Autodesk Inventor part; units mm, degrees
ref_plane "YZ Plane" through (0, 0, 0) normal (1, 0, 0) x (0, 1, 0)
ref_plane "XZ Plane" through (0, 0, 0) normal (0, 1, 0) x (-1, 0, 0)
ref_plane "XY Plane" through (0, 0, 0) normal (0, 0, 1) x (1, 0, 0)
sketch "スケッチ1" plane through (0, 0, 0) normal (0, 0, 1) x (1, 0, 0)
  line L0 (0, -4.25) -> (0.9, -4.25)
  line L1 (0.9, -4.25) -> (1.2, -3.95)
  line L2 (1.2, -3.95) -> (1.2, 1.25)
  line L3 (1.2, 1.25) -> (1.5, 1.25)
  line L4 (1.5, 1.25) -> (1.5, 1.75)
  line L5 (1.5, 1.75) -> (2.7, 1.75)
  line L6 (3, 6.95) -> (2.7, 7.25)
  line L7 (2.7, 7.25) -> (1.5, 7.25)
  line L8 (1.5, 7.25) -> (1.2, 6.95)
  line L9 (0, 7.4044) -> (0, -7.4044) construction
  line L10 (0, -4.25) -> (0, 4.25)
  line L11 (0, 4.25) -> (1.2, 4.25)
  line L12 (1.2, 4.25) -> (1.2, 6.95)
  line L13 (2.7, 1.75) -> (3, 2.05)
  line L14 (3, 2.05) -> (3, 6.95)
  point P0 (0, 0)
  point P1 (0, 0)
  dimension "d0" = 2.4
  dimension "d1" = 6
  dimension "d2" = 0.3
  dimension "d3" = 0.3
  dimension "d4" = 3
  dimension "d5" = 0.5
  dimension "d6" = 5.5
  dimension "d8" = 0.3
  dimension "d9" = 2.4
  dimension "d10" = 3
  dimension "d11" = 0.3
  dimension "d12" = 0.3
  dimension "d13" = 0.3
  dimension "d14" = 0.3
  dimension "d15" = 6
revolve "回転1" add sketch "スケッチ1" angle 360 about axis through (0, 7.4044, 0) along (0, -1, 0)
sketch "スケッチ3" plane through (0, -4.25, 0) normal (0, -1, 0) x (1, 0, 0)
  circle A0 centre (0, 0) radius 0.9
  circle A1 centre (0, 0) radius 4.1426
extrude "押し出し2" cut sketch "スケッチ3" against normal blind 3 contours A0 | A1
equation "\"d3\" = d2"
equation "\"d11\" = d8"
equation "\"d12\" = d8"
equation "\"d13\" = d12"
equation "\"d14\" = d13"
properties part number "BRU-305_5" material "ステンレス鋼 AISI 304"
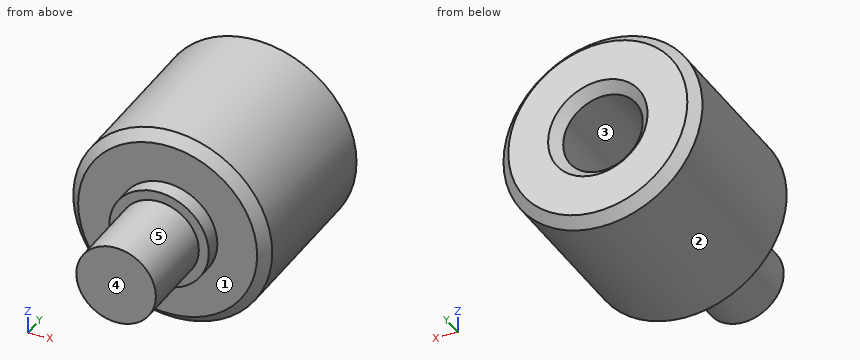
Work out the finished part from the listing and answer in its coordinate system (mm). Face numbers are marked on the shaded views. A direction names the side the tool comes from. Give positions to 0.01 mm unless a question says otherwise; leave off trailing zeros. Loops run counter-clockwise (first coordinate to the right, second up) from the corner with the lowest first, then second, coordinate; pieces in that order, holes last. Notation, with made-up numbers: (-8, -28.5) - (21, -28.5) arc R16 cw to (21, -18.5) - close; hole circle Ø6 at (-14, -40). An arc over 180 degrees is marked (long way). Answer in a Markdown table with one row per item. Add a question column.
Q1. The part is cut by section B-B (z = 0). Determine the outline of the cut face in (x, y), and give its area (3 significant figures).
Q2. The part is cut by section C-C (y = 2.75). Determine the outline of the cut face in (x, z).
Q3. Consider line 1 along Z through (x, y) = (0, 6); line 2 along Y through (x, z) = (-2.5, -0.7); line 3 along Z through (x, y) = (-0.75, 5.75). Determine where each line is inside the solid, lowest interval first.
Q4. Each of these flat-tipped pins is pushed along its axis until it touches: P1, Ø1, axis at x = -1.5, z = 0, coming from the -Y side; P2, Ø0.7, axis at x = -0.5, z = -0.5, coming from the +Y side; P3, Ø2, axis at y = 0.5, z = 1, coming from the +X side; P4, Ø2, axis at x = 2, y = 2.5, coming from the +Z side. Where does it stop, or does it pass through?
Q5. The part is cut by section D-D (y = 0). Determine the outline of the cut face in (x, z), and give its area (3 significant figures).
Q6. A tool of negligible diameter and unlimited length cuts with its end or side. For the marked faces 4 and 5, from which of +Z, -Z, +X, -X, +Y, -Y can it reach the whole face along a straight path? Write none if from no direction.
Q7. Determine the mould class of the marked faces 1, 2 and 3 for opening direction Z: released by +Z, released by -Z, zero draft, split by the parting line, or undercut.
Q8. The part is cut by section A-A (x = 0). Determine the outline of the cut face in (y, z).
Solution:
| question | item | result |
|---|---|---|
| 1 | outline | (-3, 2.05) - (-2.7, 1.75) - (-1.5, 1.75) - (-1.5, 1.25) - (-1.2, 1.25) - (-1.2, -1.25) - (1.2, -1.25) - (1.2, 1.25) - (1.5, 1.25) - (1.5, 1.75) - (2.7, 1.75) - (3, 2.05) - (3, 6.95) - (2.7, 7.25) - (1.5, 7.25) - (1.2, 6.95) - (1.2, 4.25) - (-1.2, 4.25) - (-1.2, 6.95) - (-1.5, 7.25) - (-2.7, 7.25) - (-3, 6.95) - close |
| 1 | area | 33.0 mm² |
| 2 | outline | circle Ø6 at (0, 0) |
| 3 | line 1 | z = -3 to -1.2, 1.2 to 3 |
| 3 | line 2 | y = 1.75 to 7.25 |
| 3 | line 3 | z = -2.9 to -0.94, 0.94 to 2.9 |
| 4 | P1 | stops at y = -1.25 |
| 4 | P2 | stops at y = 4.25 |
| 4 | P3 | stops at x = 1.46 |
| 4 | P4 | stops at z = 2.83 |
| 5 | outline | circle Ø2.4 at (0, 0) |
| 5 | area | 4.52 mm² |
| 6 | face 4 | +Z, -Z, +X, -X, -Y |
| 6 | face 5 | -Y |
| 7 | face 1 | zero draft |
| 7 | face 2 | split by the parting line |
| 7 | face 3 | undercut |
| 8 | outline | (-1.25, -1.2) - (1.25, -1.2) - (1.25, -1.5) - (1.75, -1.5) - (1.75, -2.7) - (2.05, -3) - (6.95, -3) - (7.25, -2.7) - (7.25, -1.5) - (6.95, -1.2) - (4.25, -1.2) - (4.25, 1.2) - (6.95, 1.2) - (7.25, 1.5) - (7.25, 2.7) - (6.95, 3) - (2.05, 3) - (1.75, 2.7) - (1.75, 1.5) - (1.25, 1.5) - (1.25, 1.2) - (-1.25, 1.2) - close |
